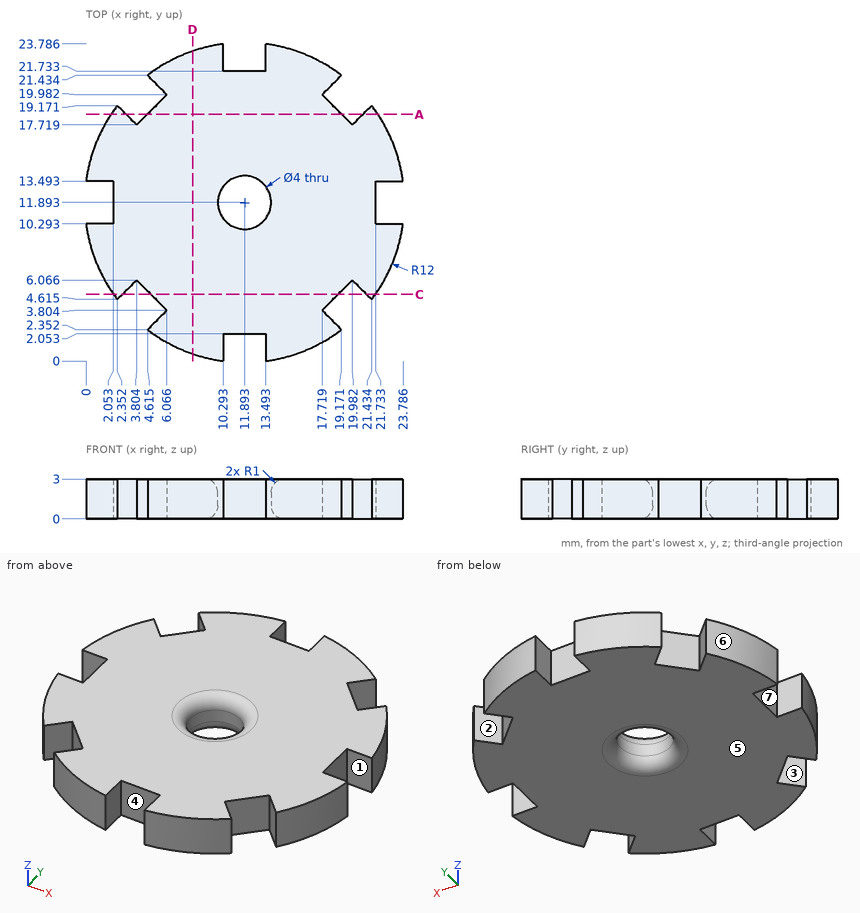
Check sheet for the drawn part. Datum: minimum x, y, z corner. Units: mm. A direction names the side the tool comes from. Round coordinates to 2 decimals unless told otherwise and drop trailing zeros. Loops run counter-clockwise (first coordinate to the right, second up) from the corner with the lowest first, then second, coordinate; pieces in that order, holes last. Notation, with made-up numbers: (47.25, -30) - (97.25, -30) arc R19 cw to (97.25, -15) - close; hole circle Ø2 at (81.25, 9). An arc over 180 degrees is marked (long way). Use one line per item in the form item = value.
1. Draft check along Y on the marked faces 4, 5, 6 and 7. Enter one of: pulls with the +Y half, pulls with the -Y half, needs draft (parallel to the pull), parting line crosses it, or undercut.
A:
face_4 = pulls with the -Y half
face_5 = needs draft
face_6 = pulls with the +Y half
face_7 = undercut
2. Section check A-A on y = 18.5. Record the cut outline in (x, z) (1 decimal).
A:
outline = (1.9, 0) - (3, 0) - (3, 3) - (1.9, 3) - close; (4.6, 0) - (19.2, 0) - (19.2, 3) - (4.6, 3) - close; (20.8, 0) - (21.9, 0) - (21.9, 3) - (20.8, 3) - close
3. Scan lines: probe 1 along Y at (x, z) = (5.75, 2.05) (1 decimal); probe 2 along Y at (x, z) = (2, 0.7) (1 decimal); probe 3 along Y at (x, z) = (22.75, 1.2) (1 decimal). Record each from-to range of solid material in increasing order.
A:
probe_1 = 1.6 to 3.5, 4.1 to 19.7, 20.3 to 22.2
probe_2 = 5.1 to 10.3, 13.5 to 18.7
probe_3 = 6.8 to 10.3, 13.5 to 17
4. Section check C-C on y = 5. Record the cut outline in (x, z) (1 decimal).
A:
outline = (2.1, 0) - (2.7, 0) - (2.7, 3) - (2.1, 3) - close; (4.9, 0) - (18.9, 0) - (18.9, 3) - (4.9, 3) - close; (21, 0) - (21.7, 0) - (21.7, 3) - (21, 3) - close
5. Section check D-D on x = 8. Record the cut outline in (y, z).
A:
outline = (0.54, 0) - (23.24, 0) - (23.24, 3) - (0.54, 3) - close
6. Access from +Z, -Z, +X, -X, +Y, -Y to the whole of each face (thin tool, end or side, straight path). Record for the marked faces 1, 2 and 3.
A:
face_1 = +Z, -Z, +X
face_2 = +Z, -Z, +Y
face_3 = +Z, -Z, -X
7. Gauge pin test, flat ends, axial feed: pin 1 Ø1.6 at (y, z) = (23, 1) entering from +X; pin 2 Ø0.9 at (x, z) = (12.5, 1.5) entering from -Y; pin 3 Ø0.6 at (y, z) = (23, 2) entering from -X (1 decimal). Record the tip position at first contact, or that the pin passes through.
A:
pin_1 = 18.04
pin_2 = 2.05
pin_3 = 6.7
